from build123d import *

# Parameters (mm, degrees)
SKETCH2_W           = 7.25
SKETCH2_H           = 4
BOSS_EXTRUDE1_DEPTH = 10
SKETCH3_R           = 0.5
CUT_EXTRUDE1_DEPTH  = 5


with BuildPart() as part:
    # Sketch2 → Boss-Extrude1 (new body)
    with BuildSketch(Plane.XY):
        with Locations((3.625, 2)):
            Rectangle(SKETCH2_W, SKETCH2_H)
    extrude(amount=BOSS_EXTRUDE1_DEPTH)

    # Sketch3 → Cut-Extrude1 (cut)
    with BuildSketch(Plane.XY.offset(10)):
        with Locations((1.125, 2)):
            Circle(SKETCH3_R)
        with Locations((2.375, 2)):
            Circle(SKETCH3_R)
        with Locations((3.625, 2)):
            Circle(SKETCH3_R)
        with Locations((4.875, 2)):
            Circle(SKETCH3_R)
        with Locations((6.125, 2)):
            Circle(SKETCH3_R)
    extrude(amount=-CUT_EXTRUDE1_DEPTH, mode=Mode.SUBTRACT)


solid = part.part
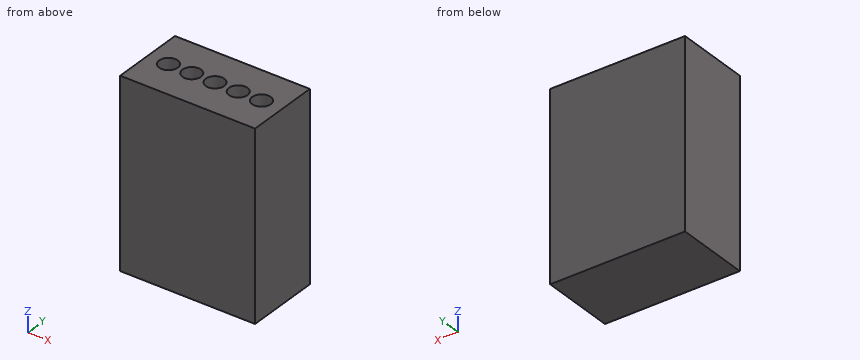
Geometry check sheet. Reference: the model listing, model coordinates, mm. Give positions to 0.01 mm unless a question says otherwise; leave off trailing zeros. Loops run counter-clockwise (first coordinate to the right, second up) from the corner with the lowest first, then second, coordinate; pieces in that order, holes last. Notation, with made-up numbers: M 86.25,-3 L 144.25,-3 A29 ccw 144.25,31 Z; hole C 31.5,52.5 d10. An arc over 180 degrees is marked long. Answer as a JSON object with one key per item and string values. Group by question number.
Item 1: Sectioned sample at A-A on z = 5.75. Record the boundary of the cut face in (x, y) (3 decimals).
Item 2: Material ranges on L1, parallel to Z at x = 4.75, y = 1.65; L2, parallel to Y at x = 5, z = 5.5; L3, parallel to Y at x = 4, z = 8.5, recorded low to high.
Item 3: Sectioned sample at B-B on x = 1. Record the boundary of the cut face in (y, z), plus the area to 3 significant figures.
Item 4: Gauge pin test, flat end, axial feed: pin 1 (0.5 mm diameter, centred on x = 5, y = 2, fed in from +Z). Record the tip position at first contact, or that the pin passes through.
Findings below:
{
 "1": {"outline": "M 0,0 L 7.25,0 L 7.25,4 L 0,4 Z; hole C 1.125,2 d1; hole C 2.375,2 d1; hole C 3.625,2 d1; hole C 4.875,2 d1; hole C 6.125,2 d1"},
 "2": {"L1": "0 to 5", "L2": "0 to 1.52, 2.48 to 4", "L3": "0 to 1.67, 2.33 to 4"},
 "3": {"outline": "M 0,0 L 4,0 L 4,10 L 2.48,10 L 2.48,5 L 1.52,5 L 1.52,10 L 0,10 Z", "area": "35.2 mm2"},
 "4": {"pin 1": "z = 5"}
}
